Here's how the part is built. I have some questions about the finished solid (model axes, mm). A direction names the side the tool comes from. Give positions to 0.01 mm unless a question says otherwise; leave off trailing zeros. Loops run counter-clockwise (first coordinate to the right, second up) from the corner with the lowest first, then second, coordinate; pieces in that order, holes last. Notation, with made-up numbers: (-35.5, 8) - (2.5, 8) arc R11 cw to (2.5, 16) - close; hole circle Ø8 at (77, 35). An arc over 180 degrees is marked (long way). Return JSON: item names as keys, results as strings. Group by question number.
(1) If we mould it in two halves opening along Z, with no side actions, what happens to faces 6 (the flat face through (-49, 2, -67)), 7 (the flat face through (34, 2, -33)), 8 (the flat face through (30.5, 2, 69)), 9 (the flat face through (67, 2, 0))? For each: released by +Z, released by -Z, zero draft, split by the parting line, or undercut.
(2) If we section it at A-A (y = 2.2): State how many separate pieces and enclosed holes the cut face has, then the cut area to 3 significant figures.
(3) If we section it at C-C (z = 8): Please give me the cut outline in (x, y), then the cut area to 3 significant figures.
(4) For P1, Ø1.5, axis at y = 1.5, z = -34, coming from the -X side; P2, Ø1.5, axis at x = -68, y = 1.5, coming from the +Z side; P3, Ø1.5, axis at y = 0.5, z = -42, coming from the +X side, each with a flat end and sliding along its axis, tell me the tip position at first contact or that it passes through.
(5) I need wall thicknesses on probe 1 along X at (y, z) = (1.75, 68.5); probe 2 along X at (y, z) = (0.25, 58). Which ranges of each line are inside material? Lowest first, please. Write a range as [from, to].
(6) If we section it at B-B (x = 11): Please give me the cut outline in (y, z).
(7) On a 3-axis mill with a long thin cutter (end or side, diameter ignored), from which of +Z, -Z, +X, -X, +Y, -Y can I reach the whole of each face in a straight line? I mean faces 1 (the flat face through (0, 2, -67)), 2 (the flat face through (-69, 2, 14.5)), 3 (the flat face through (35, 2, -35)), 4 (the flat face through (-69, 2, 30.5)), 5 (the flat face through (68, 2, 30.5)). Say none if no direction works.
```python
from build123d import *

# Parameters (mm, degrees)
BOSS_EXTRUDE1_DEPTH = 3
SKETCH2_W           = 3
SKETCH2_H           = 3
SKETCH2_H_2         = 36.5
SKETCH2_W_2         = 36.5
SKETCH2_W_3         = 29
SKETCH2_H_3         = 29
CUT_EXTRUDE2_DEPTH  = 3
SKETCH3_R           = 1.47
CUT_EXTRUDE3_DEPTH  = 3
SKETCH4_W           = 3
SKETCH4_H           = 3
CUT_EXTRUDE4_DEPTH  = 3


with BuildPart() as part:
    # Sketch1 → Boss-Extrude1 (new body)
    with BuildSketch(Plane(origin=(0, 0, 0), x_dir=(1, 0, 0), z_dir=(0, 1, 0))):
        Polygon((70, 70), (-70, 70), (0, 0), align=None)
        Polygon((0, 0), (-70, 70), (-70, -70), align=None)
        Polygon((70, -70), (0, 0), (-70, -70), align=None)
        Polygon((70, 70), (0, 0), (70, -70), align=None)
    extrude(amount=BOSS_EXTRUDE1_DEPTH)

    # Sketch2 → Cut-Extrude2 (cut)
    with BuildSketch(Plane(origin=(0, 3, 0), x_dir=(1, 0, 0), z_dir=(0, 1, 0))):
        with Locations((-68.5, 68.5)):
            Rectangle(SKETCH2_W, SKETCH2_H)
        with Locations((-68.5, 48.75)):
            Rectangle(SKETCH2_W, SKETCH2_H_2)
        with Locations((-48.75, 68.5)):
            Rectangle(SKETCH2_W_2, SKETCH2_H)
        with Locations((48.75, 68.5)):
            Rectangle(SKETCH2_W_2, SKETCH2_H)
        with Locations((68.5, 68.5)):
            Rectangle(SKETCH2_W, SKETCH2_H)
        with Locations((68.5, 48.75)):
            Rectangle(SKETCH2_W, SKETCH2_H_2)
        with Locations((68.5, -68.5)):
            Rectangle(SKETCH2_W, SKETCH2_H)
        with Locations((68.5, -48.75)):
            Rectangle(SKETCH2_W, SKETCH2_H_2)
        with Locations((48.75, -68.5)):
            Rectangle(SKETCH2_W_2, SKETCH2_H)
        with Locations((-48.75, -68.5)):
            Rectangle(SKETCH2_W_2, SKETCH2_H)
        with Locations((-68.5, -68.5)):
            Rectangle(SKETCH2_W, SKETCH2_H)
        with Locations((-68.5, -48.75)):
            Rectangle(SKETCH2_W, SKETCH2_H_2)
        with Locations((0, 68.5)):
            Rectangle(SKETCH2_W_3, SKETCH2_H)
        with Locations((0, -68.5)):
            Rectangle(SKETCH2_W_3, SKETCH2_H)
        with Locations((68.5, 0)):
            Rectangle(SKETCH2_W, SKETCH2_H_3)
        with Locations((-68.5, 0)):
            Rectangle(SKETCH2_W, SKETCH2_H_3)
    extrude(amount=-CUT_EXTRUDE2_DEPTH, mode=Mode.SUBTRACT)

    # Sketch3 → Cut-Extrude3 (cut)
    with BuildSketch(Plane(origin=(0, 3, 0), x_dir=(1, 0, 0), z_dir=(0, 1, 0))):
        with Locations((-22.5, 68.5)):
            Circle(SKETCH3_R)
        with Locations((22.5, 68.5)):
            Circle(SKETCH3_R)
        with Locations((22.5, -68.5)):
            Circle(SKETCH3_R)
        with Locations((-22.5, -68.5)):
            Circle(SKETCH3_R)
        with Locations((-68.5, 22.5)):
            Circle(SKETCH3_R)
        with Locations((-68.5, -22.5)):
            Circle(SKETCH3_R)
        with Locations((68.5, -22.5)):
            Circle(SKETCH3_R)
        with Locations((68.5, 22.5)):
            Circle(SKETCH3_R)
    extrude(amount=-CUT_EXTRUDE3_DEPTH, mode=Mode.SUBTRACT)

    # Sketch4 → Cut-Extrude4 (cut)
    with BuildSketch(Plane(origin=(0, 3, 0), x_dir=(1, 0, 0), z_dir=(0, 1, 0))):
        with Locations((35.5, 60.5)):
            Rectangle(SKETCH4_W, SKETCH4_H)
        with Locations((35.5, 33.5)):
            Rectangle(SKETCH4_W, SKETCH4_H)
    extrude(amount=-CUT_EXTRUDE4_DEPTH, mode=Mode.SUBTRACT)


solid = part.part
```
Values:
{
 "1": {"face 6": "released by -Z", "face 7": "undercut", "face 8": "zero draft", "face 9": "undercut"},
 "2": {"separate pieces": "1", "enclosed holes": "10", "area": "18,300 mm2"},
 "3": {"outline": "(-67, 0) - (67, 0) - (67, 3) - (-67, 3) - close", "area": "402 mm2"},
 "4": {"P1": "x = -67", "P2": "z = 30.5", "P3": "x = 67"},
 "5": {"probe 1": "[-30.5, -23.97], [-21.03, -14.5], [14.5, 21.03], [23.97, 30.5]", "probe 2": "[-67, 67]"},
 "6": {"outline": "(0, -67) - (3, -67) - (3, 67) - (0, 67) - close"},
 "7": {"face 1": "-Z, +Y, -Y", "face 2": "-X, +Y, -Y", "face 3": "+Y, -Y", "face 4": "+Z, -X, +Y, -Y", "face 5": "+Z, +X, +Y, -Y"}
}
